For this review, take the finished solid that the model builds, in its own axes (mm). A direction names the side the tool comes from. Coordinates: 2 decimals unless noted, no trailing zeros. Write each loop counter-clockwise with the first axis right and the second up, starting at its lowest first coordinate (ties: lowest second). Pieces come first, ordered by that corner, then holes.
1) For faces 4 (the face through (-4, 4, -41.212)), 5 (the face through (53.104, 4, 4)), 6 (the face through (97.694, 17.692, -52.259)), 7 (the face through (48, 20, 2)), list the 3-axis set-ups (+Z, -Z, +X, -X, +Y, -Y) from which the entire face can be reached by the end or side of a thin tool; tool diameter is ignored.
2) To check wall thickness, follow line 1 along Z through (x, y) = (47, 34.5); line 2 along Z through (x, y) = (0, 17); line 3 along X through (y, z) = (31.5, -7.5). State the ranges of each line that lie inside material, in increasing order.
3) We need section B-B on x = 44. Write out the cut boundary in (y, z), then the cut area to 3 significant figures.
4) Mouldability with a two-part tool opening along Z and no side actions: class faces 1 (the face through (90.6, 20, -48)), 2 (the face through (48, 18, 6)), 3 (the face through (51.2, 40, 2.5)) as pulls with the +Z half, pulls with the -Z half, needs draft (parallel to the pull), parting line crosses it, or undercut.
5) Insertion check: P1, Ø10, axis at x = 55.5, z = -29, coming from the +Y side; P2, Ø3, axis at y = 23.5, z = 0.5, coming from the +X side; P3, Ø3, axis at y = 5.5, z = 4, coming from the -X side; P4, Ø3, axis at x = 94.1, z = 0, coming from the -Y side. Each pin has a flat end and moves straight along its axis. Give the tip position at first contact, or say it passes through.
6) We need section C-C on y = 24.5. Write out the cut boundary in (x, z).
7) We need section A-A on z = -36.5. Write out the cut boundary in (x, y).
from build123d import *
from build123d.topology import SkipClean

# Parameters (mm, degrees)
SKETCH1_R           = 1.65
BOSS_EXTRUDE1_DEPTH = 40
BOSS_EXTRUDE2_START = 4
SKETCH2_R           = 1.65
BOSS_EXTRUDE2_DEPTH = 4
SKETCH3_W           = 15.5
SKETCH3_H           = 8.5
CUT_EXTRUDE1_DEPTH  = 4
SKETCH5_W           = 13
SKETCH5_H           = 8
CUT_EXTRUDE2_DEPTH  = 4
SKETCH6_W           = 13
SKETCH6_H           = 8
CUT_EXTRUDE3_DEPTH  = 4


with BuildPart() as part:
    # Sketch1 → Boss-Extrude1 (new body)
    with BuildSketch(Plane(origin=(0, 0, 0), x_dir=(1, 0, 0), z_dir=(0, 1, 0))):
        with BuildLine():
            Line((2, 54.54), (92.1, 54.54))
            ThreePointArc((92.1, 54.54), (97.756854249, 52.196854249), (100.1, 46.54))
            Line((100.1, 46.54), (100.1, 2))
            ThreePointArc((100.1, 2), (97.756854249, -3.656854249), (92.1, -6))
            Line((92.1, -6), (2, -6))
            ThreePointArc((2, -6), (-3.656854249, -3.656854249), (-6, 2))
            Line((-6, 2), (-6, 46.54))
            ThreePointArc((-6, 46.54), (-3.656854249, 52.196854249), (2, 54.54))
        make_face()
        with Locations(Location((0, 48.54, 0), (0, 0, 270))):
            Circle(SKETCH1_R, mode=Mode.SUBTRACT)
        with Locations(Location((0, 0, 0), (0, 0, 270))):
            Circle(SKETCH1_R, mode=Mode.SUBTRACT)
        with Locations(Location((94.1, 48.54, 0), (0, 0, 270))):
            Circle(SKETCH1_R, mode=Mode.SUBTRACT)
        with Locations(Location((94.1, 0, 0), (0, 0, 270))):
            Circle(SKETCH1_R, mode=Mode.SUBTRACT)
        Polygon((-2, 45.04), (3.5, 45.04), (3.5, 50.54), (90.6, 50.54), (90.6, 45.04), (96.1, 45.04), (96.1, 3.5), (90.6, 3.5), (90.6, -2), (3.5, -2), (3.5, 3.5), (-2, 3.5), align=None, mode=Mode.SUBTRACT)
    extrude(amount=BOSS_EXTRUDE1_DEPTH)

    # Sketch2 → Boss-Extrude2 (add)
    with SkipClean():  # the faces are left unmerged after this step: merging them gives an invalid solid
        with BuildSketch(Plane.XZ.offset(BOSS_EXTRUDE2_START)):
            with BuildLine():
                Line((100.1, -46.54), (100.1, -2))
                ThreePointArc((100.1, -2), (97.756854249, 3.656854249), (92.1, 6))
                Line((92.1, 6), (2, 6))
                ThreePointArc((2, 6), (-3.656854249, 3.656854249), (-6, -2))
                Line((-6, -2), (-6, -46.54))
                ThreePointArc((-6, -46.54), (-3.656854249, -52.196854249), (2, -54.54))
                Line((2, -54.54), (92.1, -54.54))
                ThreePointArc((92.1, -54.54), (97.756854249, -52.196854249), (100.1, -46.54))
            make_face()
            with Locations(Location((94.1, 0, 0), (0, 0, 270))):
                Circle(SKETCH2_R, mode=Mode.SUBTRACT)
            with Locations(Location((94.1, -48.54, 0), (0, 0, 270))):
                Circle(SKETCH2_R, mode=Mode.SUBTRACT)
            with Locations(Location((0, -48.54, 0), (0, 0, 270))):
                Circle(SKETCH2_R, mode=Mode.SUBTRACT)
            with Locations(Location((0, 0, 0), (0, 0, 270))):
                Circle(SKETCH2_R, mode=Mode.SUBTRACT)
        extrude(amount=-BOSS_EXTRUDE2_DEPTH)

    # Sketch3 → Cut-Extrude1 (cut)
    with SkipClean():  # the faces are left unmerged after this step: merging them gives an invalid solid
        with BuildSketch(Plane.XY.offset(6)):
            with Locations((45.353986939, 4.25)):
                Rectangle(SKETCH3_W, SKETCH3_H)
        extrude(amount=-CUT_EXTRUDE1_DEPTH, mode=Mode.SUBTRACT)

    # Sketch5 → Cut-Extrude2 (cut)
    with SkipClean():  # the faces are left unmerged after this step: merging them gives an invalid solid
        with BuildSketch(Plane.ZY.offset(6)):
            with Locations((-34.712384261, 4)):
                Rectangle(SKETCH5_W, SKETCH5_H)
        extrude(amount=-CUT_EXTRUDE2_DEPTH, mode=Mode.SUBTRACT)

    # Sketch6 → Cut-Extrude3 (cut)
    with SkipClean():  # the faces are left unmerged after this step: merging them gives an invalid solid
        with BuildSketch(Plane.XY.offset(6)):
            with Locations((26.272328528, 4)):
                Rectangle(SKETCH6_W, SKETCH6_H)
        extrude(amount=-CUT_EXTRUDE3_DEPTH, mode=Mode.SUBTRACT)


solid = part.part
Result:
1. face 4: -X
1. face 5: +Z
1. face 6: -Z, +X, +Y, -Y
1. face 7: +Y
2. line 1: z = -54.54 to -50.54, 2 to 6
2. line 2: z = -54.29 to -50.19, -46.89 to -45.04, -3.5 to -1.65, 1.65 to 5.75
2. line 3: x = -6 to -2, 96.1 to 100.1
3. outline: (-4, -54.54) - (40, -54.54) - (40, -50.54) - (0, -50.54) - (0, 6) - (-4, 6) - close; (8.5, 2) - (40, 2) - (40, 6) - (8.5, 6) - close
3. area: 528 mm2
4. face 1: undercut
4. face 2: pulls with the +Z half
4. face 3: needs draft
5. P1: stops at y = 0
5. P2: stops at x = 100.04
5. P3: stops at x = -4.61
5. P4: passes through
6. outline: (-6, -46.54) arc R8 ccw to (2, -54.54) - (92.1, -54.54) arc R8 ccw to (100.1, -46.54) - (100.1, -2) arc R8 ccw to (92.1, 6) - (2, 6) arc R8 ccw to (-6, -2) - close; hole (-2, -45.04) - (3.5, -45.04) - (3.5, -50.54) - (90.6, -50.54) - (90.6, -45.04) - (96.1, -45.04) - (96.1, -3.5) - (90.6, -3.5) - (90.6, 2) - (3.5, 2) - (3.5, -3.5) - (-2, -3.5) - close; hole circle Ø3.3 at (0, -48.54); hole circle Ø3.3 at (0, 0); hole circle Ø3.3 at (94.1, -48.54); hole circle Ø3.3 at (94.1, 0)
7. outline: (-6, -4) - (100.1, -4) - (100.1, 40) - (96.1, 40) - (96.1, 0) - (-6, 0) - close; (-6, 8) - (-2, 8) - (-2, 40) - (-6, 40) - close
